Geometry check sheet. Reference: drawing and pictorial views, mm from the part's lowest x, y, z. A direction names the side the tool comes from. Give positions to 0.01 mm unless a question says otherwise; leave off trailing zeros. Write each loop counter-clockwise with the first axis right and the second up, starting at its lowest first coordinate (ties: lowest second). Pieces come first, ordered by that corner, then holes. Notation, with made-up numbers: M -9,-13.75 L 36,-13.75 A25 ccw 36,12.25 Z; hole C 64,-23 d11. An arc over 180 degrees is marked long. One line per item, written item: value. Start each with the question number.
1. Gauge pin test, flat ends, axial feed: pin 1 (4 mm diameter, centred on x = 35.5, z = 3.85, fed in from -Y); pin 2 (5 mm diameter, centred on x = 17.5, z = 48.5, fed in from +Y); pin 3 (3.5 mm diameter, centred on y = 27.5, z = 7.5, fed in from -X). Record the tip position at first contact, or that the pin passes through.
2. Scan lines: line 1 (Z direction, x = 35, y = 26) (1 decimal); line 2 (Y direction, x = 6.5, z = 44). Record each from-to range of solid material in increasing order.
3. Tool access check on the marked faces 1 and 2. Record the directions out of +Z, -Z, +X, -X, +Y, -Y that give a thin tool (end or side, any length) a straight path to the whole face; none if there is none.
4. Release check for a two-part mould opening along Z. For the marked faces 3 and 4 record: pulls with the +Z half, pulls with the -Z half, needs draft (parallel to the pull), parting line crosses it, or undercut.
5. Cross-section at A-A on y = 27.5. Record the cut outline in (x, z) (1 decimal).
6. Cross-section at C-C on y = 6.5. Record the cut outline in (x, z).
7. Cross-section at D-D on x = 35.5. Record the cut outline in (y, z).
8. Cross-section at B-B on x = 4. Record the cut outline in (y, z).
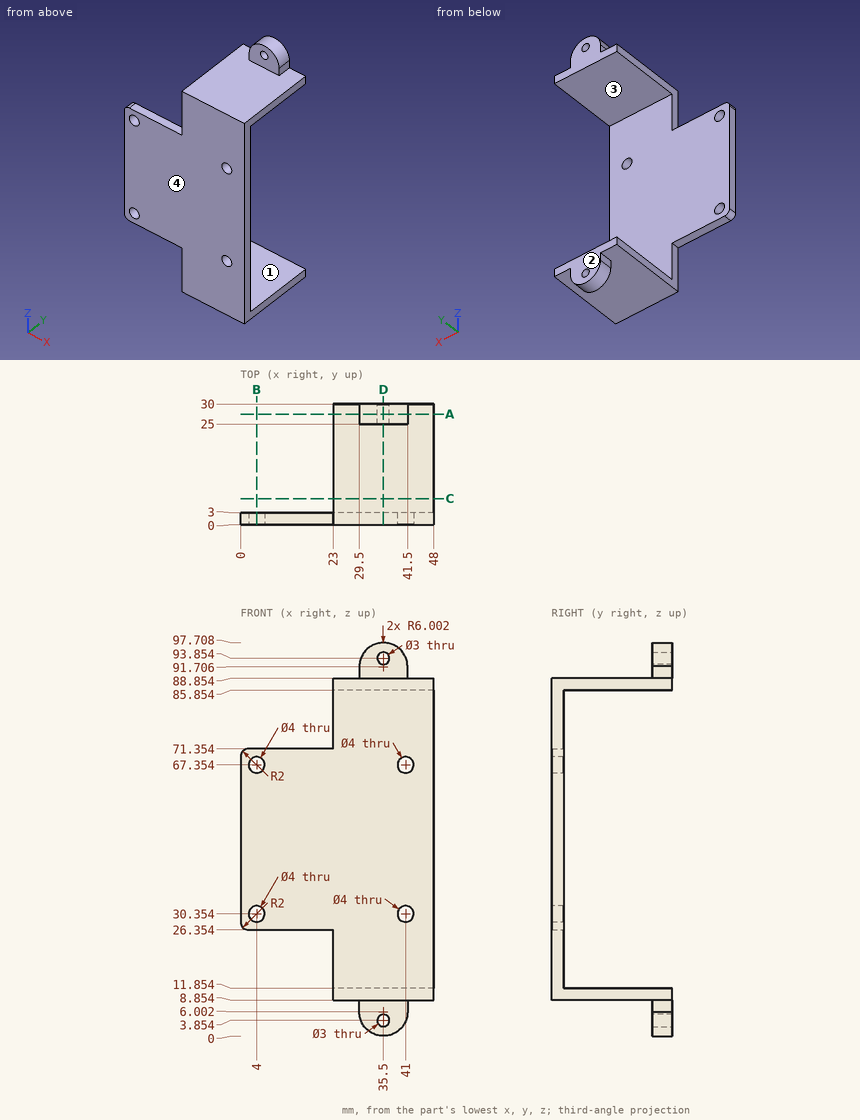
Report:
1. pin 1: stops at y = 25
1. pin 2: stops at y = 3
1. pin 3: stops at x = 23
2. line 1: z = 0 to 2.4, 5.3 to 11.9, 85.9 to 92.4, 95.3 to 97.7
2. line 2: y = 0 to 3
3. face 1: +X, -X, +Y
3. face 2: +Z, -Z, +X, -X, +Y
4. face 3: undercut
4. face 4: needs draft
5. outline: M 23,8.9 L 29.5,8.9 L 29.5,5.9 A6 ccw 41.5,5.9 L 41.5,8.9 L 48,8.9 L 48,11.9 L 23,11.9 Z; M 23,85.9 L 48,85.9 L 48,88.9 L 41.5,88.9 L 41.5,91.9 A6 ccw 29.5,91.9 L 29.5,88.9 L 23,88.9 Z; hole C 35.5,3.9 d3; hole C 35.5,93.9 d3
6. outline: M 23,8.85 L 48,8.85 L 48,11.85 L 23,11.85 Z; M 23,85.85 L 48,85.85 L 48,88.85 L 23,88.85 Z
7. outline: M 0,8.85 L 25,8.85 L 25,5.35 L 30,5.35 L 30,11.85 L 3,11.85 L 3,85.85 L 30,85.85 L 30,92.35 L 25,92.35 L 25,88.85 L 0,88.85 Z; M 25,0 L 30,0 L 30,2.35 L 25,2.35 Z; M 25,95.35 L 30,95.35 L 30,97.71 L 25,97.71 Z
8. outline: M 0,26.35 L 3,26.35 L 3,28.35 L 0,28.35 Z; M 0,32.35 L 3,32.35 L 3,65.35 L 0,65.35 Z; M 0,69.35 L 3,69.35 L 3,71.35 L 0,71.35 Z
